```python
from build123d import *

# Parameters (mm, degrees)
SKETCH1_W               = 121
SKETCH1_H               = 60
SKETCH1_R               = 5
SKETCH1_R_2             = 3.25
SKETCH1_R_3             = 2.83
SKETCH1_R_4             = 1.6
SKETCH1_W_2             = 8.7
SKETCH1_H_2             = 3.4
BOSS_EXTRUDE1_DEPTH     = 4
SKETCH2_W               = 4
SKETCH2_H               = 60
BOSS_EXTRUDE2_DEPTH     = 4
CUT_EXTRUDE2_DEPTH      = 85.599054368
CUT_EXTRUDE2_DEPTH_BACK = 85.599054368
SKETCH3_W               = 3.4
SKETCH3_H               = 8.7


with BuildPart() as part:
    # Sketch1 → Boss-Extrude1 (new body)
    with BuildSketch(Plane.XY):
        with Locations((-18.5, 0)):
            Rectangle(SKETCH1_W, SKETCH1_H)
        with Locations((-46, 0)):
            Circle(SKETCH1_R, mode=Mode.SUBTRACT)
        with Locations((-12.5, 17)):
            Circle(SKETCH1_R_2, mode=Mode.SUBTRACT)
        with Locations((16, -24)):
            Circle(SKETCH1_R_3, mode=Mode.SUBTRACT)
        with Locations((-5, 0)):
            Circle(SKETCH1_R_4, mode=Mode.SUBTRACT)
        with Locations((-59.65, -13.3)):
            Rectangle(SKETCH1_W_2, SKETCH1_H_2, mode=Mode.SUBTRACT)
        with Locations((33.55, -13.3)):
            Rectangle(SKETCH1_W_2, SKETCH1_H_2, mode=Mode.SUBTRACT)
    extrude(amount=BOSS_EXTRUDE1_DEPTH)

    # Sketch2 → Boss-Extrude2 (add)
    with BuildSketch(Plane.XY):
        with Locations((44, 0)):
            Rectangle(SKETCH2_W, SKETCH2_H)
    extrude(amount=BOSS_EXTRUDE2_DEPTH)

    # Sketch3 → Cut-Extrude2 (cut, two sides: drawn at the far end of the back side and taken through both)
    with BuildSketch(Plane.XY.offset(-CUT_EXTRUDE2_DEPTH_BACK)):
        with Locations((40.3, 21.65)):
            Rectangle(SKETCH3_W, SKETCH3_H)
        with Locations((40.3, -21.65)):
            Rectangle(SKETCH3_W, SKETCH3_H)
    extrude(amount=CUT_EXTRUDE2_DEPTH + CUT_EXTRUDE2_DEPTH_BACK, mode=Mode.SUBTRACT)


solid = part.part
```
Here's how the part is built. I have some questions about the finished solid (model axes, mm). A direction names the side the tool comes from. Round coordinates to 2 decimals unless told otherwise and drop trailing zeros. Order: outer loops, then holes, each group sorted by start corner. A loop starts at its lowest first (then second) coordinate and runs counter-clockwise, first axis right, second up. Notation, with made-up numbers: M 17.25,-12 L 46.25,-12 A36 cw 46.25,24 Z; hole C 28,32 d7. An arc over 180 degrees is marked long. Answer in a Markdown table with one row per item.
Item 1: Imagine slicing it at D-D, the plane y = 0. Write out the boundary of the cut face in (x, z), and give its area (3 significant figures).
A:
| item | result |
|---|---|
| outline | M -79,0 L -51,0 L -51,4 L -79,4 Z; M -41,0 L -6.6,0 L -6.6,4 L -41,4 Z; M -3.4,0 L 46,0 L 46,4 L -3.4,4 Z |
| area | 447 mm2 |
Item 2: Thinking about a two-plate mould opening in X: for faces 1 (the face through (38.6, 22, 2)), 2 (the face through (-17, 0, 4)), which applies, +X half, -X half, draft (parallel to the pull), parting line (faces both ways), or undercut?
A:
| item | result |
|---|---|
| face 1 | undercut |
| face 2 | draft |
Item 3: For faces 3 (the face through (-17, -30, 2)), 4 (the face through (40, 26, 2)), which set-ups out of +Z, -Z, +X, -X, +Y, -Y let a thin tool reach every point of the face, with its end or its side?
A:
| item | result |
|---|---|
| face 3 | +Z, -Z, +X, -X, -Y |
| face 4 | +Z, -Z |
Item 4: Imagine slicing it at B-B, the plane x = -12.5. Write out the boundary of the cut face in (y, z), and give its area (3 significant figures).
A:
| item | result |
|---|---|
| outline | M -30,0 L 13.75,0 L 13.75,4 L -30,4 Z; M 20.25,0 L 30,0 L 30,4 L 20.25,4 Z |
| area | 214 mm2 |
Item 5: Imagine slicing it at A-A, the plane y = -19. Write out the boundary of the cut face in (x, z).
A:
| item | result |
|---|---|
| outline | M -79,0 L 38.6,0 L 38.6,4 L -79,4 Z; M 42,0 L 46,0 L 46,4 L 42,4 Z |
Item 6: Imagine slicing it at C-C, the plane z = 1.35. State how many separate pieces and enclosed holes the cut face has, and give its area (3 significant figures).
A:
| item | result |
|---|---|
| separate pieces | 1 |
| enclosed holes | 8 |
| area | 7,240 mm2 |
Item 7: If I drill on L1, parallel to X at y = -19, z = 0.25; L2, parallel to X at y = 19, z = 0.55; L3, parallel to Y at x = -46, z = 1.15, over which ranges is the centre line in solid material (lowest first)? Write a range as from..to.
A:
| item | result |
|---|---|
| L1 | x = -79..38.6, 42..46 |
| L2 | x = -79..-15.06, -9.94..38.6, 42..46 |
| L3 | y = -30..-5, 5..30 |
